Autodesk Inventor part; units mm, degrees
ref_plane "YZ Plane" through (0, 0, 0) normal (1, 0, 0) x (0, 1, 0)
ref_plane "XZ Plane" through (0, 0, 0) normal (0, 1, 0) x (-1, 0, 0)
ref_plane "XY Plane" through (0, 0, 0) normal (0, 0, 1) x (1, 0, 0)
sketch "Sketch1" plane through (0, 0, 0) normal (0, 1, 0) x (-1, 0, 0)
  line L0 (20, 45) -> (-20, 45)
  line L1 (-20, 45) -> (-20, -45)
  line L2 (-20, -45) -> (20, -45)
  line L3 (20, 45) -> (-20, -45) construction
  line L4 (-20, 45) -> (20, -45) construction
  arc A0 (-20, -45) -> (20, -45) centre (0, -45) ccw
  line L5 (20, 45) -> (20, -45)
  line L6 (-20, -45) -> (-50, -45)
  line L7 (-50, -45) -> (-50, 45)
  line L8 (-50, 45) -> (-20, 45)
  line L9 (-20, 45) -> (-20, -45)
  point P0 (0, 0)
  dimension "d0" = 40
  dimension "d1" = 90
  dimension "d26" = 30
extrude "Extrusion1" add sketch "Sketch1" along normal blind 3.6
sketch "Sketch2" plane through (0, 3.6, 0) normal (0, 1, 0) x (1, 0, 0)
  arc A0 (20, 45) -> (-20, 45) centre (0, 45) ccw
  circle A1 centre (0, 45) radius 5.15
  point P0 (0, 0)
  dimension "d4" = 10.3
extrude "Extrusion2" cut sketch "Sketch2" against normal blind 3.6
fillet "Fillet1" radius 4 4 edges at (-20, 1.8, -45) (50, 1.8, 45) (-20, 1.8, 45) (20, 1.8, -45)
chamfer "Chamfer1" distance 20 angle 45 1 edges at (50, 1.8, -45)
fillet "Fillet2" radius 10 2 edges at (30, 1.8, -45) (50, 1.8, -25)
sketch "Sketch5" plane through (0, 0, 0) normal (0, -1, 0) x (1, 0, 0)
  circle A0 centre (25, -41.5) radius 1.625
  circle A1 centre (46.5, -21.5) radius 1.625
  circle A2 centre (46.5, 41.5) radius 1.625
  circle A3 centre (-16.5, -23.5) radius 1.625
  line L0 (25.8579, -45) -> (23.6643, -45)
  line L1 (50, 41) -> (50, -20.8579)
  line L2 (-20, -45) -> (-20, 41)
  line L3 (-16, 45) -> (46, 45)
  circle A4 centre (-16.5, 41.5) radius 1.625
  point P0 (0, 0)
  dimension "d31" = 3.25
  dimension "d32" = 3.25
  dimension "d34" = 3.25
  dimension "d35" = 3.25
  dimension "d36" = 3.5
  dimension "d37" = 3.5
  dimension "d38" = 3.5
  dimension "d40" = 25
  dimension "d41" = 20
  dimension "d42" = 3.5
  dimension "d43" = 3.5
  dimension "d48" = 3.25
  dimension "d49" = 3.5
  dimension "d50" = 3.5
  dimension "d52" = 65
extrude "Extrusion5" cut sketch "Sketch5" against normal blind 10
properties part number "p1"
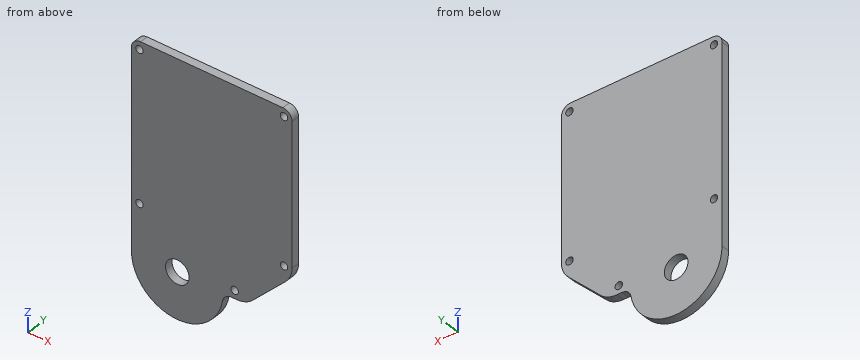
Design review of the part built by this model. Coordinates are the model's own, in mm. Coordinates: 2 decimals unless noted, no trailing zeros. Order: outer loops, then holes, each group sorted by start corner. A loop starts at its lowest first (then second) coordinate and runs counter-clockwise, first axis right, second up.
Item 1: Take a section at A-A, the plane y = 3. Write out the cut boundary in (x, z) (3 decimals), then the cut area to 3 significant figures.
Item 2: Take a section at B-B, the plane z = -56. Write out the cut boundary in (x, y), then the cut area to 3 significant figures.
Item 3: For line 1 (Z direction, x = -16.5, y = 1.8) (3 decimals); line 2 (Z direction, x = 46.5, y = 2.2) (3 decimals); line 3 (Z direction, x = 25, y = 2.5) (3 decimals), list the stretches that pass through material, from the lowest coordinate up.
Item 4: For pin 1 Ø3 at (x, z) = (46.5, -21.5) entering from +Y; pin 2 Ø1 at (x, y) = (-9.5, 3) entering from -Z; pin 3 Ø1.1 at (x, y) = (25.5, 2.5) entering from -Z, all flat-tipped, find the tip position at first contact; note any pin that passes through.
The answers:
1. outline: (-20, -45) arc R20 ccw to (19.72, -48.333) arc R4 cw to (23.664, -45) - (25.858, -45) arc R10 ccw to (32.929, -42.071) - (47.071, -27.929) arc R10 ccw to (50, -20.858) - (50, 41) arc R4 ccw to (46, 45) - (-16, 45) arc R4 ccw to (-20, 41) - close; hole circle Ø3.25 at (-16.5, -23.5); hole circle Ø3.25 at (-16.5, 41.5); hole circle Ø10.3 at (0, -45); hole circle Ø3.25 at (25, -41.5); hole circle Ø3.25 at (46.5, -21.5); hole circle Ø3.25 at (46.5, 41.5)
1. area: 6,590 mm2
2. outline: (-16.7, 0) - (16.7, 0) - (16.7, 3.6) - (-16.7, 3.6) - close
2. area: 120 mm2
3. line 1: z = -56.303 to -25.125, -21.875 to 39.875, 43.125 to 44.969
3. line 2: z = -28.5 to -23.125, -19.875 to 39.875, 43.125 to 44.969
3. line 3: z = -45 to -43.125, -39.875 to 45
4. pin 1: passes through
4. pin 2: stops at z = -62.86
4. pin 3: stops at z = -45
